The listing builds one solid part. Answer for the finished solid, in the listing's coordinates (mm). A direction names the side the tool comes from. Give positions to 0.01 mm unless a question says otherwise; leave off trailing zeros. Write each loop counter-clockwise with the first axis right and the second up, starting at its lowest first coordinate (ties: lowest second). Pieces come first, ordered by that corner, then holes. Notation, with made-up numbers: (33, -39.5) -> (67, -39.5) arc R30 ccw to (67, -2.5) -> close; hole circle Ø6 at (-24.5, 5.25). An arc over 180 degrees is marked (long way). Put each result on its own line as item: value. Start each with the question number.
1) For a pull along Y with two mould halves and no side action, classify faces 1 (the flat face through (1, -34.793, 301)), 2 (the flat face through (0, -33.523, 301)), 3 (the flat face through (-12, -9, 0)) as released by +Y, released by -Y, zero draft, split by the parting line, or undercut.
2) A cutting plane is placed at A-A (x = -6.5). Write down the section's boundary in (y, z), then the cut area to 3 significant figures.
3) A cutting plane is placed at B-B (z = 514). Write down the section's boundary in (x, y).
4) Find the intervals of material crossed by line 1 along Y through (x, z) = (5.5, 93); line 2 along X through (y, z) = (-34.45, 571.5); line 3 along X through (y, z) = (8, 115), in increasing order. Write a range as from..to.
5) For faces 4 (the flat face through (11.959, -10, 301)), 5 (the flat face through (-12, -9, 609.6)), determine the directions among +Z, -Z, +X, -X, +Y, -Y from which every point of the face is accessible in a straight line to the end or side of a thin tool.
6) Flat-ended cylindrical pins translate along their axes: pin 1 Ø4.5 at (y, z) = (-9.39, 584.2) entering from -X; pin 2 Ø5.5 at (x, z) = (0.53, 114.3) entering from -Y. Find the tip coordinate at first contact, or state that the pin passes through.
Autodesk Inventor part; units mm, degrees
ref_plane "YZ Plane" through (0, 0, 0) normal (1, 0, 0) x (0, 1, 0)
ref_plane "XZ Plane" through (0, 0, 0) normal (0, 1, 0) x (-1, 0, 0)
ref_plane "XY Plane" through (0, 0, 0) normal (0, 0, 1) x (1, 0, 0)
sketch "Sketch1" plane through (0, 0, 0) normal (0, 0, 1) x (1, 0, 0)
  line L0 (-12.1708, 16.0073) -> (13.2292, 16.0073)
  line L1 (13.2292, 16.0073) -> (13.2292, -34.7927)
  line L2 (13.2292, -34.7927) -> (-12.1708, -34.7927)
  line L3 (-12.1708, -34.7927) -> (-12.1708, 16.0073)
  line L4 (11.9592, 14.7373) -> (-10.9008, 14.7373)
  line L5 (-10.9008, 14.7373) -> (-10.9008, -33.5227)
  line L6 (-10.9008, -33.5227) -> (11.9592, -33.5227)
  line L7 (11.9592, -33.5227) -> (11.9592, 14.7373)
  point P0 (0, 0)
  dimension "d0" = 25.4
  dimension "d1" = 50.8
  dimension "d2" = 1.27
extrude "Extrusion1" add sketch "Sketch1" along normal blind 609.6
sketch "Sketch2" plane through (-12.1708, 16.0073, 0) normal (0, 1, 0) x (1, 0, 0)
  circle A0 centre (12.7, -12.7) radius 1.7272
  line L0 (25.4, 0) -> (0, 0)
  line L1 (0, 0) -> (0, -609.6)
  point P0 (12.1708, 0)
  dimension "d5" = 3.4544
  dimension "d6" = 12.7
  dimension "d7" = 12.7
extrude "Extrusion2" cut sketch "Sketch2" against normal through all
pattern_linear "Rectangular Pattern1" count 61 spacing 25.4 along (0, 0, 1) of "Extrusion2"
sketch "Sketch6" plane through (-12.1708, -34.7927, 0) normal (-1, 0, 0) x (0, 0, 1)
  circle A0 centre (203.2, 25.4) radius 2.3813
  circle A1 centre (177.8, 25.4) radius 2.3813
  circle A2 centre (152.4, 25.4) radius 2.3813
  line L0 (152.4, 25.4) -> (203.2, 25.4)
  line L1 (0, 50.8) -> (0, 0)
  line L2 (0, 50.8) -> (609.6, 50.8)
  circle A3 centre (596.9, 25.4) radius 2.3813
  circle A4 centre (584.2, 25.4) radius 2.3813
  circle A5 centre (571.5, 25.4) radius 2.3813
  line L3 (571.5, 25.4) -> (596.9, 25.4)
  line L4 (609.6, 50.8) -> (609.6, 0)
  point P0 (0, 34.7927)
  dimension "d38" = 4.7625
  dimension "d39" = 50.8
  dimension "d41" = 25.4
  dimension "d43" = 152.4
  dimension "d44" = 4.7625
  dimension "d45" = 25.4
  dimension "d46" = 25.4
  dimension "d47" = 12.7
extrude "Extrusion6" cut sketch "Sketch6" against normal through all
sketch "Sketch7" plane through (-12.1708, -34.7927, 0) normal (-1, 0, 0) x (0, 0, 1)
  circle A0 centre (63.5, 25.4) radius 14.2875
  line L0 (0, 50.8) -> (0, 0)
  line L1 (0, 0) -> (609.6, 0)
  point P0 (0, 34.7927)
  dimension "d50" = 63.5
  dimension "d51" = 25.4
  dimension "d52" = 28.575
extrude "Extrusion7" cut sketch "Sketch7" against normal through all
equation "\"d3\" = d13"
equation "\"d10\" = d14"
equation "\"d13\" = 609.6"
equation "\"d14\" = d13"
properties part number "Long bar 3- VersaFrame"
Reply:
1. face 1: released by -Y
1. face 2: undercut
1. face 3: zero draft
2. outline: (-34.79, 0) -> (-33.52, 0) -> (-33.52, 609.6) -> (-34.79, 609.6) -> close; (14.74, 0) -> (16.01, 0) -> (16.01, 609.6) -> (14.74, 609.6) -> close
2. area: 1,550 mm2
3. outline: (-12.17, -34.79) -> (13.23, -34.79) -> (13.23, 16.01) -> (-12.17, 16.01) -> close; hole (-10.9, -33.52) -> (11.96, -33.52) -> (11.96, 14.74) -> (-10.9, 14.74) -> close
4. line 1: y = -34.79..-33.52, 14.74..16.01
4. line 2: x = -12.17..-1.2, 2.26..13.23
4. line 3: x = -12.17..-10.9, 11.96..13.23
5. face 4: +Z, -Z
5. face 5: +Z, +X, -X, +Y, -Y
6. pin 1: passes through
6. pin 2: stops at y = -34.79
